```python
from build123d import *

# Parameters (mm, degrees)
SKETCH1_R           = 12.15
SKETCH1_R_2         = 16.15
BOSS_EXTRUDE1_DEPTH = 5.2
CUT_EXTRUDE1_DEPTH  = 86.894153614
FILLET1_R           = 30
CHAMFER1_SIZE       = 1
SKETCH2_R           = 14.75534968
SKETCH2_R_2         = 10
SKETCH2_R_3         = 19.025242353
SKETCH2_R_4         = 14
BOSS_EXTRUDE2_DEPTH = 0.6


with BuildPart() as part:
    # Sketch1 → Boss-Extrude1 (new body)
    with BuildSketch(Plane(origin=(0, 0, 0), x_dir=(1, 0, 0), z_dir=(0, 1, 0))):
        with BuildLine():
            Line((50.6952797, -21), (62.125, -21))
            ThreePointArc((62.125, -21), (83.125, 0), (62.125, 21))
            Line((62.125, 21), (50.6952797, 21))
            ThreePointArc((50.6952797, 21), (44.646090821, 13.026866227), (35.106613419, 10))
            Line((35.106613419, 10), (-35.106613419, 10))
            ThreePointArc((-35.106613419, 10), (-44.646090821, 13.026866227), (-50.6952797, 21))
            Line((-50.6952797, 21), (-62.125, 21))
            ThreePointArc((-62.125, 21), (-83.125, 0), (-62.125, -21))
            Line((-62.125, -21), (-50.6952797, -21))
            ThreePointArc((-50.6952797, -21), (-44.646090821, -13.026866227), (-35.106613419, -10))
            Line((-35.106613419, -10), (35.106613419, -10))
            ThreePointArc((35.106613419, -10), (44.646090821, -13.026866227), (50.6952797, -21))
        make_face()
        with Locations(Location((-62.125, 0, 0), (0, 0, 270))):
            Circle(SKETCH1_R, mode=Mode.SUBTRACT)
        with Locations(Location((62.125, 0, 0), (0, 0, 270))):
            Circle(SKETCH1_R_2, mode=Mode.SUBTRACT)
    extrude(amount=BOSS_EXTRUDE1_DEPTH)

    # Sketch4 → Cut-Extrude1 (cut, through all)
    with BuildSketch(Plane(origin=(0, 5.2, 0), x_dir=(1, 0, 0), z_dir=(0, 1, 0))):
        with BuildLine():
            Line((-62.125, 16.5), (-40.410985901, 16.5))
            Line((-40.410985901, 16.5), (-43.407950199, 33.342917206))
            Line((-43.407950199, 33.342917206), (-92.984497382, 23.090976894))
            Line((-92.984497382, 23.090976894), (-92.984497382, -9.501012459))
            Line((-92.984497382, -9.501012459), (-86.710921967, -27.097626428))
            Line((-86.710921967, -27.097626428), (-50.736883487, -31.973137348))
            Line((-50.736883487, -31.973137348), (-37.899444956, -29.584754809))
            Line((-37.899444956, -29.584754809), (-38.970543198, -16.5))
            Line((-38.970543198, -16.5), (-62.125, -16.5))
            ThreePointArc((-62.125, -16.5), (-78.625, 0), (-62.125, 16.5))
        make_face()
    extrude(amount=-CUT_EXTRUDE1_DEPTH, mode=Mode.SUBTRACT)

    # Fillet1
    # the kernel refuses this fillet: 30 mm, written as the material it takes off along each edge
    with BuildSketch(Plane(origin=(50.6952797, -28.574300751, -21), x_dir=(1, 0, 0), z_dir=(0, 1, 0))) as fillet1_piece_1:
        with BuildLine():
            CenterArc((14.667456891, -29.824772619), FILLET1_R, 96.195688925, 34.34815674)
            ThreePointArc((-4.833435899, -7.027510056), (-1.956106094, -3.830558257), (0, 0))
            Line((0, 0), (11.4297203, 0))
        make_face()
    extrude(amount=62.348601502, mode=Mode.SUBTRACT)
    with BuildSketch(Plane(origin=(50.6952797, -28.574300751, 21), x_dir=(1, 0, 0), z_dir=(0, 1, 0))) as fillet1_piece_2:
        with BuildLine():
            CenterArc((14.667456891, 29.824772619), FILLET1_R, 229.456154336, 34.34815674)
            ThreePointArc((-4.833435899, 7.027510056), (-1.956106094, 3.830558257), (0, 0))
            Line((0, 0), (11.4297203, 0))
        make_face()
    extrude(amount=62.348601502, mode=Mode.SUBTRACT)
    with BuildSketch(Plane(origin=(-48.253657182, 31.64326437, -16.5), x_dir=(-1, 0, 0), z_dir=(0, -1, 0))) as fillet1_piece_3:
        with BuildLine():
            CenterArc((10.577305748, -30), FILLET1_R, 90, 30.643820853)
            ThreePointArc((-4.713681591, -4.189426465), (-2.15539677, -2.321365496), (0, 0))
            Line((0, 0), (10.577305748, 0))
        make_face()
    extrude(amount=58.086528739, mode=Mode.SUBTRACT)
    with BuildSketch(Plane(origin=(-48.253657182, 31.64326437, 16.5), x_dir=(0.7474496885574631, 0, -0.6643184199428399), z_dir=(0, -1, 0))) as fillet1_piece_4:
        with BuildLine():
            CenterArc((12.023548711, -29.450189698), FILLET1_R, 100.986236803, 30.643820853)
            Line((-7.906003887, -7.026699042), (0, 0))
            ThreePointArc((0, 0), (3.153176503, -0.30323414), (6.306353006, 0))
        make_face()
    extrude(amount=58.086528739, mode=Mode.SUBTRACT)

    # Chamfer1
    # the kernel refuses this chamfer: 1 mm, written as the material it takes off along each edge
    with BuildSketch(Plane(origin=(62.125, 5.2, 0), x_dir=(-0.12235070165055903, 0, 0.9924869297908239), z_dir=(-0.9924869297908239, 0, -0.12235070165055903))) as chamfer1_piece_1:
        Polygon((21, -CHAMFER1_SIZE), (21 - CHAMFER1_SIZE, 0), (21, 0), align=None)
    revolve(axis=Axis((62.125, 5.2, 0), (0, 1, 0)), revolution_arc=194.055575488, mode=Mode.SUBTRACT)
    with BuildSketch(Plane(origin=(35.106613419, 5.2, -26.545750746), x_dir=(0.6500297596931421, 0, 0.7599087520967739), z_dir=(0.7599087520967739, 0, -0.6500297596931421))) as chamfer1_piece_2:
        Polygon((16.545750746 + CHAMFER1_SIZE, 0), (16.545750746, CHAMFER1_SIZE), (16.545750746, 0), align=None)
    revolve(axis=Axis((35.106613419, 5.2, -26.545750746), (0, -1, 0)), revolution_arc=40.543845664, mode=Mode.SUBTRACT)
    with BuildSketch(Plane(origin=(35.106613419, 5.2, -10), x_dir=(0, 0, 1), z_dir=(-1, 0, 0)), Plane(origin=(-35.106613419, 5.2, 10), x_dir=(0, 0, -1), z_dir=(1, 0, 0))) as chamfer1_piece_3:
        Polygon((CHAMFER1_SIZE, 0), (0, -CHAMFER1_SIZE), (0, 0), align=None)
    extrude(amount=70.213226838, mode=Mode.SUBTRACT)
    with BuildSketch(Plane(origin=(-62.125, 5.2, 0), x_dir=(0, 0, 1), z_dir=(1, 0, 0))) as chamfer1_piece_4:
        Polygon((16.5 - CHAMFER1_SIZE, 0), (16.5, CHAMFER1_SIZE), (16.5, 0), align=None)
    revolve(axis=Axis((-62.125, 5.2, 0), (0, -1, 0)), revolution_arc=180, mode=Mode.SUBTRACT)
    with BuildSketch(Plane(origin=(-62.125, 5.2, -16.5), x_dir=(0, 0, 1), z_dir=(1, 0, 0)), Plane(origin=(-58.83096293, 5.2, 16.5), x_dir=(0, 0, -1), z_dir=(-1, 0, 0))) as chamfer1_piece_5:
        Polygon((CHAMFER1_SIZE, 0), (0, CHAMFER1_SIZE), (0, 0), align=None)
    extrude(amount=3.29403707, mode=Mode.SUBTRACT)
    with BuildSketch(Plane(origin=(-35.106613419, 5.2, 26.545750746), x_dir=(-0.5096995779497587, 0, -0.8603524511720982), z_dir=(-0.8603524511720982, 0, 0.5096995779497587))) as chamfer1_piece_6:
        Polygon((16.545750746 + CHAMFER1_SIZE, 0), (16.545750746, CHAMFER1_SIZE), (16.545750746, 0), align=None)
    revolve(axis=Axis((-35.106613419, 5.2, 26.545750746), (0, -1, 0)), revolution_arc=30.643820853, mode=Mode.SUBTRACT)
    with BuildSketch(Plane(origin=(-62.125, 5.2, 0), x_dir=(0, 0, 1), z_dir=(-1, 0, 0))) as chamfer1_piece_7:
        Polygon((12.15 + CHAMFER1_SIZE, 0), (12.15, -CHAMFER1_SIZE), (12.15, 0), align=None)
    revolve(axis=Axis((-62.125, 5.2, 0), (0, 1, 0)), mode=Mode.SUBTRACT)
    with BuildSketch(Plane(origin=(62.125, 5.2, 0), x_dir=(0, 0, 1), z_dir=(-1, 0, 0))) as chamfer1_piece_8:
        Polygon((16.15 + CHAMFER1_SIZE, 0), (16.15, -CHAMFER1_SIZE), (16.15, 0), align=None)
    revolve(axis=Axis((62.125, 5.2, 0), (0, 1, 0)), mode=Mode.SUBTRACT)
    with BuildSketch(Plane(origin=(-35.106613419, 5.2, -26.545750746), x_dir=(0, 0, 1), z_dir=(1, 0, 0))) as chamfer1_piece_9:
        Polygon((16.545750746 + CHAMFER1_SIZE, 0), (16.545750746, CHAMFER1_SIZE), (16.545750746, 0), align=None)
    revolve(axis=Axis((-35.106613419, 5.2, -26.545750746), (0, -1, 0)), revolution_arc=30.643820853, mode=Mode.SUBTRACT)
    with BuildSketch(Plane(origin=(35.106613419, 5.2, 26.545750746), x_dir=(0, 0, -1), z_dir=(-1, 0, 0))) as chamfer1_piece_10:
        Polygon((16.545750746 + CHAMFER1_SIZE, 0), (16.545750746, CHAMFER1_SIZE), (16.545750746, 0), align=None)
    revolve(axis=Axis((35.106613419, 5.2, 26.545750746), (0, -1, 0)), revolution_arc=40.543845664, mode=Mode.SUBTRACT)
    with BuildSketch(Plane(origin=(65.362736591, 5.2, -8.824772619), x_dir=(0.14849692395329253, 0, 0.9889128695574804), z_dir=(0.9889128695574804, 0, -0.14849692395329253))) as chamfer1_piece_11:
        Polygon((30, CHAMFER1_SIZE), (30 - CHAMFER1_SIZE, 0), (30, 0), align=None)
    revolve(axis=Axis((65.362736591, 5.2, -8.824772619), (0, -1, 0)), revolution_arc=49.083676808, mode=Mode.SUBTRACT)
    with BuildSketch(Plane(origin=(65.362736591, 5.2, 8.824772619), x_dir=(-0.6500297596931309, 0, -0.7599087520967833), z_dir=(-0.7599087520967833, 0, 0.6500297596931309))) as chamfer1_piece_12:
        Polygon((30, CHAMFER1_SIZE), (30 - CHAMFER1_SIZE, 0), (30, 0), align=None)
    revolve(axis=Axis((65.362736591, 5.2, 8.824772619), (0, -1, 0)), revolution_arc=49.083676808, mode=Mode.SUBTRACT)
    with BuildSketch(Plane(origin=(-58.83096293, 5.2, -13.5), x_dir=(0, 0, 1), z_dir=(-1, 0, 0))) as chamfer1_piece_13:
        Polygon((30 - CHAMFER1_SIZE, 0), (30, -CHAMFER1_SIZE), (30, 0), align=None)
    revolve(axis=Axis((-58.83096293, 5.2, -13.5), (0, 1, 0)), revolution_arc=30.643820853, mode=Mode.SUBTRACT)
    with BuildSketch(Plane(origin=(-58.83096293, 5.2, 13.5), x_dir=(0.5096995779497117, 0, -0.8603524511721262), z_dir=(0.8603524511721262, 0, 0.5096995779497117))) as chamfer1_piece_14:
        Polygon((30 - CHAMFER1_SIZE, 0), (30, -CHAMFER1_SIZE), (30, 0), align=None)
    revolve(axis=Axis((-58.83096293, 5.2, 13.5), (0, 1, 0)), revolution_arc=30.643820853, mode=Mode.SUBTRACT)

    # Sketch2 → Boss-Extrude2 (add)
    # profile 1 of 2: a face of its own
    with BuildSketch(Plane.XZ):
        with Locations((-62.125, 0)):
            Circle(SKETCH2_R)
        with Locations(Location((-62.125, 0, 0), (0, 0, 270))):
            Circle(SKETCH2_R_2, mode=Mode.SUBTRACT)
    # profile 2 of 2: a face of its own
    with BuildSketch(Plane.XZ):
        with Locations((62.125, 0)):
            Circle(SKETCH2_R_3)
        with Locations(Location((62.125, 0, 0), (0, 0, 270))):
            Circle(SKETCH2_R_4, mode=Mode.SUBTRACT)
    extrude(amount=-BOSS_EXTRUDE2_DEPTH)


solid = part.part
```
Could you check a few things on this model? Use its own coordinates, in mm. A direction names the side the tool comes from. Give positions to 0.01 mm unless a question says otherwise; leave off trailing zeros. Loops run counter-clockwise (first coordinate to the right, second up) from the corner with the lowest first, then second, coordinate; pieces in that order, holes last. Notation, with made-up numbers: (52.25, 78) - (69.25, 78) arc R31 cw to (69.25, 114) - close; hole circle Ø6 at (27.5, 58). An arc over 180 degrees is marked (long way). Answer in a Markdown table with one row per item. Add a question column.
Q1. If we section it at B-B (y = 1.8): State how many separate pieces and enclosed holes the cut face has, plus the area to 3 significant figures.
Q2. We'd pull the mould along X, two halves only. Please class faces 5 (the face through (-50.795, 2.129, 15.404)), 6 (the face through (-77.79, 5.03, 0.34)), 7 (the face through (-60, 2, 16.5)): +X half, -X half, draft (parallel to the pull), parting line (faces both ways), or undercut.
Q3. For pin 1 (2 mm diameter, centred on x = 39, y = 3.5, fed in from -Z); pin 2 (1.6 mm diameter, centred on x = -60.5, y = 1.5, fed in from -Z); pin 3 (1.6 mm diameter, centred on x = -59.5, y = 3, fed in from +Z), each with a flat end and sliding along its axis, tell me the tip position at first contact or that it passes through.
Q4. Which directions (+Z, -Z, +X, -X, +Y, -Y) give clear straight access to the entire face, cutting with the end or side of a thin tool? Please do faces 1 (the face through (62, 0.6, 14.4)), 2 (the face through (2, 5.2, 1)), 3 (the face through (53.347, 2.071, 18.664)), 4 (the face through (0, 2, -10)).
Q5. If we section it at C-C (x = -16): List the corners of the cut face in (y, z) for me.
Q6. If we section it at A-A (z = 0): List the corners of the cut face in (x, y) for me (3 decimals).
Q7. Please list where these lines run through material, in increasing order: L1, parallel to X at y = 0.25, z = 0 (3 decimals); L2, parallel to X at y = 2.1, z = 0 (3 decimals); L3, parallel to Z at x = -58, y = 1.35. Write a range as from..to.
The answers:
| question | item | result |
|---|---|---|
| 1 | separate pieces | 1 |
| 1 | enclosed holes | 2 |
| 1 | area | 2,840 mm^2 |
| 2 | face 5 | undercut |
| 2 | face 6 | -X half |
| 2 | face 7 | draft |
| 3 | pin 1 | stops at z = -10.74 |
| 3 | pin 2 | stops at z = -16.5 |
| 3 | pin 3 | stops at z = 16.5 |
| 4 | face 1 | +Y |
| 4 | face 2 | +Z, -Z, +X, -X, +Y |
| 4 | face 3 | +Z, +Y, -Y |
| 4 | face 4 | -Z, +Y, -Y |
| 5 | outline | (0, -10) - (4.2, -10) - (5.2, -9) - (5.2, 9) - (4.2, 10) - (0, 10) - close |
| 6 | outline | (-78.625, 0) - (-72.125, 0) - (-72.125, 0.6) - (-74.275, 0.6) - (-74.275, 4.2) - (-75.275, 5.2) - (-77.625, 5.2) - (-78.625, 4.2) - close; (-52.125, 0) - (48.125, 0) - (48.125, 0.6) - (45.975, 0.6) - (45.975, 4.2) - (44.975, 5.2) - (-48.975, 5.2) - (-49.975, 4.2) - (-49.975, 0.6) - (-52.125, 0.6) - close; (76.125, 0) - (83.125, 0) - (83.125, 4.2) - (82.125, 5.2) - (79.275, 5.2) - (78.275, 4.2) - (78.275, 0.6) - (76.125, 0.6) - close |
| 7 | L1 | x = -78.625..-72.125, -52.125..48.125, 76.125..83.125 |
| 7 | L2 | x = -78.625..-74.275, -49.975..45.975, 78.275..83.125 |
| 7 | L3 | z = -16.49..-11.43, 11.43..16.49 |
